Source: CAD feature listing. Evaluate the final solid. Frame: model axes, mm. Face numbers are marked on the shaded views. A direction names the side the tool comes from. Round coordinates to 2 decimals unless told otherwise and drop trailing zeros. Write each loop counter-clockwise with the first axis right and the second up, starting at its lowest first coordinate (ties: lowest second). Pieces come first, ordered by that corner, then holes. Notation, with made-up numbers: (-25.5, 9.5) -> (11.5, 9.5) arc R29 ccw to (11.5, 33.5) -> close; hole circle Ø10 at (7, -1). An arc over 180 degrees is marked (long way). Put each result on its own line as item: value.
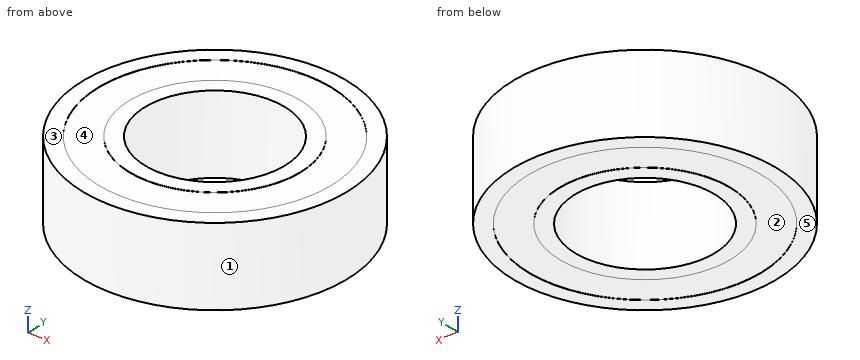
```python
from build123d import *

# Parameters (mm, degrees)
BOSS_EXTRUDE1_DEPTH        = 2.5
BOSS_EXTRUDE1_DEPTH_BACK   = 2.5
SKETCH1_R                  = 8.5
SKETCH1_R_2                = 7.5
BOSS_EXTRUDE1_2_DEPTH      = 2.5
BOSS_EXTRUDE1_2_DEPTH_BACK = 2.5
SKETCH1_R_3                = 5.5
SKETCH1_R_4                = 4.5
BOSS_EXTRUDE2_DEPTH        = 2.484375
BOSS_EXTRUDE2_DEPTH_BACK   = 2.484375
SKETCH1_3_R                = 7.5
SKETCH1_3_R_2              = 5.5


with BuildPart() as part:
    # Sketch1 → Boss-Extrude1 (new, two sides: drawn at the far end of the back side and taken through both)
    with BuildSketch(Plane.XY.offset(-BOSS_EXTRUDE1_DEPTH_BACK)):
        Circle(SKETCH1_R)
        Circle(SKETCH1_R_2, mode=Mode.SUBTRACT)
    extrude(amount=BOSS_EXTRUDE1_DEPTH + BOSS_EXTRUDE1_DEPTH_BACK)



with BuildPart() as body_2:
    # Sketch1 → Boss-Extrude1 2 (new, two sides: drawn at the far end of the back side and taken through both)
    with BuildSketch(Plane.XY.offset(-BOSS_EXTRUDE1_2_DEPTH_BACK)):
        Circle(SKETCH1_R_3)
        Circle(SKETCH1_R_4, mode=Mode.SUBTRACT)
    extrude(amount=BOSS_EXTRUDE1_2_DEPTH + BOSS_EXTRUDE1_2_DEPTH_BACK)


with BuildPart() as part_1:
    add(part.part)

    add(body_2.part)  # Boss-Extrude2 merges body 2
    # Sketch1_3 → Boss-Extrude2 (add, two sides: drawn at the far end of the back side and taken through both)
    with BuildSketch(Plane.XY.offset(-BOSS_EXTRUDE2_DEPTH_BACK)):
        Circle(SKETCH1_3_R)
        Circle(SKETCH1_3_R_2, mode=Mode.SUBTRACT)
    extrude(amount=BOSS_EXTRUDE2_DEPTH + BOSS_EXTRUDE2_DEPTH_BACK)


solid = part_1.part
```
Q1. Cut plane C-C on z = -1.9. Output: boundary loops of the cut face in (x, y), and give its area (3 significant figures).
Ans:
outline: circle Ø17 at (0, 0); hole circle Ø9 at (0, 0)
area: 163 mm^2
Q2. Draft query along Y for the marked faces 1, 2 and 3. Return one class per face: +Y half, -Y half, draft (parallel to the pull), parting line (faces both ways), or undercut.
Ans:
face 1: parting line
face 2: undercut
face 3: draft
Q3. Pin query (flat end, axial travel): pin 1 (2 mm diameter, centred on x = 3, z = 1, fed in from +Y); pin 2 (1.5 mm diameter, centred on y = 2.5, z = 2, fed in from -X); pin 3 (2 mm diameter, centred on x = 5, z = 1.5, fed in from -Y). Return the tip coordinate at first contact, or that it passes through.
Ans:
pin 1: stops at y = 8.26
pin 2: stops at x = -8.32
pin 3: stops at y = -7.5
Q4. Reachability of the marked faces 4 and 5 from +Z, -Z, +X, -X, +Y, -Y: full face, straight path, thin tool, end or side. Return the list, or none.
Ans:
face 4: +Z
face 5: -Z, +X, -X, +Y, -Y
Q5. Material intervals for line 1 (Y direction, x = 0, z = -1.3); line 2 (Z direction, x = -4.75, y = -4.25); line 3 (Y direction, x = 0.75, z = -1.55), sorted ascending. Write a range as [from, to].
Ans:
line 1: y = [-8.5, -4.5], [4.5, 8.5]
line 2: z = [-2.48, 2.48]
line 3: y = [-8.47, -4.44], [4.44, 8.47]
